The listing builds one solid part. Answer for the finished solid, in the listing's coordinates (mm). A direction names the side the tool comes from. Round coordinates to 2 decimals unless told otherwise and drop trailing zeros. Write each loop counter-clockwise with the first axis right and the second up, starting at its lowest first coordinate (ties: lowest second). Pieces come first, ordered by that corner, then holes.
from build123d import *

# Parameters (mm, degrees)
SKETCH_W     = 20
SKETCH_H     = 83.26
SKETCH_R     = 1.75
SKETCH_R_2   = 2.25
PAD_DEPTH    = 5
SKETCH001_W  = 5
SKETCH001_H  = 63.26
PAD001_DEPTH = 5


with BuildPart() as part:
    # Sketch → Pad (new body)
    with BuildSketch(Plane.XY):
        with Locations((-48.41, -7.5)):
            Rectangle(SKETCH_W, SKETCH_H)
        with Locations((-48.41, -24.13)):
            Circle(SKETCH_R, mode=Mode.SUBTRACT)
        with Locations((-48.41, 24.13)):
            Circle(SKETCH_R, mode=Mode.SUBTRACT)
        with Locations((-48.41, -39.13)):
            Circle(SKETCH_R_2, mode=Mode.SUBTRACT)
    extrude(amount=PAD_DEPTH)

    # Sketch001 → Pad001 (new body)
    with BuildSketch(Plane.XY.offset(5)):
        with Locations((-40.91, 2.5)):
            Rectangle(SKETCH001_W, SKETCH001_H)
        with Locations((-55.91, 2.5)):
            Rectangle(SKETCH001_W, SKETCH001_H)
    extrude(amount=PAD001_DEPTH)


solid = part.part
1. A tool of negligible diameter and unlimited length cuts with its end or side. For faces 1 (the face through (-49, -7, 0)), 2 (the face through (-53.41, 2, 7)), 3 (the face through (-41, -29.13, 7)), from which of +Z, -Z, +X, -X, +Y, -Y can it reach the whole face along a straight path? Write none if from no direction.
Geometry says:
face 1: -Z, +X, -X, +Y, -Y
face 2: +Z, +Y, -Y
face 3: +Z, +X, -X, -Y
2. Section A-A on z = 9 is taken. Determine the outline of the cut face in (x, y).
Geometry says:
outline: (-58.41, -29.13) - (-53.41, -29.13) - (-53.41, 34.13) - (-58.41, 34.13) - close; (-43.41, -29.13) - (-38.41, -29.13) - (-38.41, 34.13) - (-43.41, 34.13) - close
3. Section B-B on x = -48.41 is taken. Determine the outline of the cut face in (y, z).
Geometry says:
outline: (-49.13, 0) - (-41.38, 0) - (-41.38, 5) - (-49.13, 5) - close; (-36.88, 0) - (-25.88, 0) - (-25.88, 5) - (-36.88, 5) - close; (-22.38, 0) - (22.38, 0) - (22.38, 5) - (-22.38, 5) - close; (25.88, 0) - (34.13, 0) - (34.13, 5) - (25.88, 5) - close
4. For a pull along X with two mould halves and no side action, classify faces 4 (the face through (-41, 3, 10)), 5 (the face through (-38.41, -8, 5)), 6 (the face through (-43.41, 2, 7)) as released by +X, released by -X, zero draft, split by the parting line, or undercut.
Geometry says:
face 4: zero draft
face 5: released by +X
face 6: undercut
5. Section C-C on y = -24.13 is taken. Determine the outline of the cut face in (x, z).
Geometry says:
outline: (-58.41, 0) - (-50.16, 0) - (-50.16, 5) - (-53.41, 5) - (-53.41, 10) - (-58.41, 10) - close; (-46.66, 0) - (-38.41, 0) - (-38.41, 10) - (-43.41, 10) - (-43.41, 5) - (-46.66, 5) - close
6. Straight lines are drawn through the part: line 1 along Y through (x, z) = (-48.41, 1.35); line 2 along X through (y, z) = (-14, 7.25); line 3 along Y through (x, z) = (-47.25, 1.25). For each, find the intervals that lie inside material, in ascending order.
Geometry says:
line 1: y = -49.13 to -41.38, -36.88 to -25.88, -22.38 to 22.38, 25.88 to 34.13
line 2: x = -58.41 to -53.41, -43.41 to -38.41
line 3: y = -49.13 to -41.06, -37.2 to -25.44, -22.82 to 22.82, 25.44 to 34.13
7. Section D-D on z = 1.75 is taken. Determine the outline of the cut face in (x, y), plus the area to 3 significant figures.
Geometry says:
outline: (-58.41, -49.13) - (-38.41, -49.13) - (-38.41, 34.13) - (-58.41, 34.13) - close; hole circle Ø4.5 at (-48.41, -39.13); hole circle Ø3.5 at (-48.41, -24.13); hole circle Ø3.5 at (-48.41, 24.13)
area: 1,630 mm2
8. Given pin 1 (6 mm diameter, centred on x = -47.5, y = 2, fed in from +Z); pin 2 (4 mm diameter, centred on x = -40, z = 8, fed in from -Y), each flat-ended and moving along its own axis, determine where each tip first touches the part or whether it passes through.
Geometry says:
pin 1: stops at z = 5
pin 2: stops at y = -29.13
